Verification items for the finished model (mm, model axes). Coordinates: 2 decimals unless noted, no trailing zeros. Loops run counter-clockwise (first coordinate to the right, second up) from the corner with the lowest first, then second, coordinate; pieces in that order, holes last. Notation, with made-up numbers: (87, 78.25) -> (121, 78.25) arc R24 cw to (121, 111.25) -> close; hole circle Ø2 at (-29, 76.25). An arc over 180 degrees is marked (long way). Answer as a JSON object with one key per item and string values. Group by question number.
Q1. Cross-section at D-D on z = 38.3. Record the boundary of the cut face in (x, y), and give its area (3 significant figures).
Q2. Cross-section at C-C on x = 9. Record the boundary of the cut face in (y, z), and give its area (3 significant figures).
Q3. Cross-section at B-B on z = 27.5. Record the boundary of the cut face in (x, y).
Q4. Scan lines: L1, parallel to X at y = -1.15, z = 17.5; L2, parallel to X at y = -2.5, z = 24.5; L3, parallel to X at y = -1.8, z = 28.5. Record each from-to range of solid material in increasing order.
Q5. Cross-section at A-A on y = -2.2. Record the boundary of the cut face in (x, z).
Q6. Gauge pin test, flat ends, axial feed: pin 1 Ø5.5 at (x, z) = (-36.75, 38.3) entering from -Y; pin 2 Ø0.8 at (y, z) = (-0.5, 24) entering from +X; pin 3 Ø4.5 at (x, z) = (36.75, 38.3) entering from -Y. Record the tip position at first contact, or that the pin passes through.
```python
from build123d import *

# Parameters (mm, degrees)
SKETCH033_R     = 1.75
SKETCH033_R_2   = 7.75
SKETCH033_R_3   = 3.6
PAD001_DEPTH    = 3
CHAMFER001_SIZE = 2
CHAMFER002_SIZE = 1.4
SKETCH035_R     = 9
POCKET008_DEPTH = 1.501
POCKET009_DEPTH = 1


with BuildPart() as part:
    # Sketch033 → Pad001 (new body)
    with BuildSketch(Plane.XZ):
        with BuildLine():
            Line((-34.303718, 43.4), (34.303711, 43.4))
            ThreePointArc((42.299997, 35.643765), (39.873715, 41.142392), (34.303711, 43.4))
            Line((42.299997, 35.643765), (43.05, 11.043791))
            ThreePointArc((35.053716, 2.8), (40.796116, 5.230006), (43.05, 11.043791))
            Line((35.053716, 2.8), (-35.053716, 2.8))
            ThreePointArc((-43.05, 11.043802), (-40.79612, 5.23001), (-35.053716, 2.8))
            Line((-43.05, 11.043802), (-42.300003, 35.643776))
            ThreePointArc((-34.303718, 43.4), (-39.873717, 41.142396), (-42.300003, 35.643776))
        make_face()
        with Locations((-36.75, 38.3)):
            Circle(SKETCH033_R, mode=Mode.SUBTRACT)
        with Locations((36.75, 38.3)):
            Circle(SKETCH033_R, mode=Mode.SUBTRACT)
        with Locations((-38, 8.3)):
            Circle(SKETCH033_R, mode=Mode.SUBTRACT)
        with Locations((38, 8.3)):
            Circle(SKETCH033_R, mode=Mode.SUBTRACT)
        with Locations((-31, 21.5)):
            Circle(SKETCH033_R_2, mode=Mode.SUBTRACT)
        with Locations((31, 25.5)):
            Circle(SKETCH033_R_3, mode=Mode.SUBTRACT)
        with BuildLine():
            Line((-14, 33.75), (14, 33.75))
            ThreePointArc((16, 31.75), (15.414214, 33.164214), (14, 33.75))
            Line((16, 31.75), (16, 19.25))
            ThreePointArc((14, 17.25), (15.414214, 17.835786), (16, 19.25))
            Line((14, 17.25), (-14, 17.25))
            ThreePointArc((-16, 19.25), (-15.414214, 17.835786), (-14, 17.25))
            Line((-16, 19.25), (-16, 31.75))
            ThreePointArc((-14, 33.75), (-15.414214, 33.164214), (-16, 31.75))
        make_face(mode=Mode.SUBTRACT)
    extrude(amount=PAD001_DEPTH)

    # Chamfer001
    chamfer001_edges = [part.edges().sort_by_distance(p)[0] for p in [
        (0, -3, 33.75),
    ]]
    chamfer(chamfer001_edges, length=CHAMFER001_SIZE)

    # Chamfer002
    chamfer002_edges = [part.edges().sort_by_distance(p)[0] for p in [
        (-39.75, -3, 8.3),
        (-38.5, -3, 38.3),
        (36.25, -3, 8.3),
        (35, -3, 38.3),
    ]]
    chamfer(chamfer002_edges, length=CHAMFER002_SIZE)

    # Sketch035 → Pocket008 (cut, through all)
    with BuildSketch(Plane.XZ.offset(1.5)):
        with Locations((-31, 21.5)):
            Circle(SKETCH035_R)
    extrude(amount=POCKET008_DEPTH, mode=Mode.SUBTRACT)

    # Sketch036 → Pocket009 (cut)
    with BuildSketch(Plane.XZ):
        with BuildLine():
            ThreePointArc((30, 20.25), (29.25, 19.5), (30, 18.75))
            Line((30, 18.75), (32, 18.75))
            ThreePointArc((32, 18.75), (32.75, 19.5), (32, 20.25))
            Line((30, 20.25), (32, 20.25))
        make_face()
    extrude(amount=POCKET009_DEPTH, mode=Mode.SUBTRACT)


solid = part.part
```
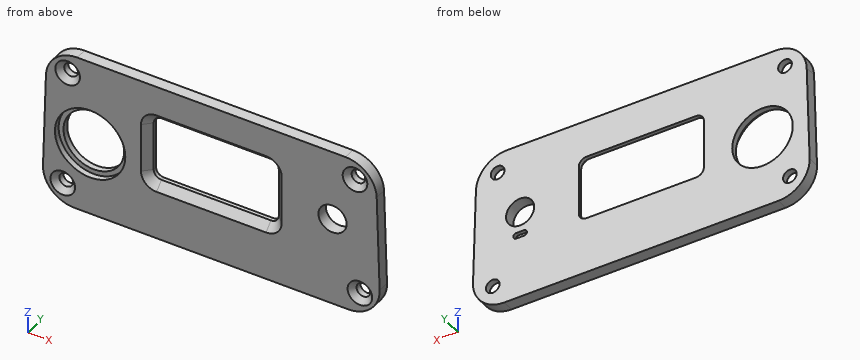
Computed values:
{
 "1": {"outline": "(-41.76, -3) -> (-39.9, -3) -> (-38.5, -1.6) -> (-38.5, 0) -> (-41.76, 0) -> close; (-35, -1.6) -> (-33.6, -3) -> (33.6, -3) -> (35, -1.6) -> (35, 0) -> (-35, 0) -> close; (38.5, -1.6) -> (39.9, -3) -> (41.76, -3) -> (41.76, 0) -> (38.5, 0) -> close", "area": "226 mm²"},
 "2": {"outline": "(-3, 2.8) -> (0, 2.8) -> (0, 17.25) -> (-1, 17.25) -> (-3, 15.25) -> close; (-3, 35.75) -> (-1, 33.75) -> (0, 33.75) -> (0, 43.4) -> (-3, 43.4) -> close", "area": "68.3 mm²"},
 "3": {"outline": "(-42.55, -3) -> (-37.71, -3) -> (-37.71, -1.5) -> (-35.91, -1.5) -> (-35.91, 0) -> (-42.55, 0) -> close; (-26.09, -1.5) -> (-24.29, -1.5) -> (-24.29, -3) -> (-18, -3) -> (-16, -1) -> (-16, 0) -> (-26.09, 0) -> close; (16, -1) -> (18, -3) -> (28.01, -3) -> (28.01, 0) -> (16, 0) -> close; (33.99, -3) -> (42.55, -3) -> (42.55, 0) -> (33.99, 0) -> close"},
 "4": {"L1": "x = -42.85 to -37.64, -24.36 to -15.25, 15.25 to 42.85", "L2": "x = -42.64 to -39.49, -22.51 to -17.5, 17.5 to 27.54, 34.46 to 42.64", "L3": "x = -42.52 to -36.66, -25.34 to -16.8, 16.8 to 29.01, 32.99 to 42.52"},
 "5": {"outline": "(-43.05, 11.04) arc R8 ccw to (-35.05, 2.8) -> (35.05, 2.8) arc R8 ccw to (43.05, 11.04) -> (42.3, 35.64) arc R8 ccw to (34.3, 43.4) -> (-34.3, 43.4) arc R8 ccw to (-42.3, 35.64) -> close; hole circle Ø4.7 at (-38, 8.3); hole circle Ø18 at (-31, 21.5); hole circle Ø4.7 at (-36.75, 38.3); hole (-17.2, 19.25) arc R3.2 ccw to (-14, 16.05) -> (14, 16.05) arc R3.2 ccw to (17.2, 19.25) -> (17.2, 31.75) arc R3.2 ccw to (14, 34.95) -> (-14, 34.95) arc R3.2 ccw to (-17.2, 31.75) -> close; hole circle Ø7.2 at (31, 25.5); hole circle Ø4.7 at (36.75, 38.3); hole circle Ø4.7 at (38, 8.3)"},
 "6": {"pin 1": "stops at y = -2.6", "pin 2": "stops at x = 42.67", "pin 3": "stops at y = -2.1"}
}
